The listing builds one solid part. Answer for the finished solid, in the listing's coordinates (mm). Face numbers are marked on the shaded views. A direction names the side the tool comes from. Coordinates: 2 decimals unless noted, no trailing zeros. Write each loop counter-clockwise with the first axis right and the second up, starting at its lowest first coordinate (ties: lowest second). Pieces come first, ordered by that corner, then holes. Notation, with made-up numbers: M 11,20 L 31,20 A4 cw 31,26 Z; hole C 3,58 d7. An arc over 180 degrees is marked long. Answer as a JSON object with one key per item and string values. Group by question number.
from build123d import *

# Parameters (mm, degrees)
SKETCH2_W           = 62
SKETCH2_H           = 49
BOSS_EXTRUDE2_DEPTH = 16
SKETCH3_W           = 60.436043862
SKETCH3_H           = 47.036060162
CUT_EXTRUDE2_DEPTH  = 15.492
SKETCH4_W           = 26
SKETCH4_H           = 26
CUT_EXTRUDE3_DEPTH  = 1.014
SKETCH6_W           = 11.5
SKETCH6_H           = 10
CUT_EXTRUDE4_DEPTH  = 1.014
FILLET3_R           = 1
SKETCH8_W           = 33.330843918
SKETCH8_H           = 11.266105729
BOSS_EXTRUDE3_DEPTH = 5.586
SKETCH9_W           = 2.5
SKETCH9_H           = 30.963135996
CUT_EXTRUDE5_DEPTH  = 13.714


with BuildPart() as part:
    # Sketch2 → Boss-Extrude2 (new body)
    with BuildSketch(Plane(origin=(0, 0, 0), x_dir=(1, 0, 0), z_dir=(0, 1, 0))):
        Rectangle(SKETCH2_W, SKETCH2_H)
    extrude(amount=BOSS_EXTRUDE2_DEPTH)

    # Sketch3 → Cut-Extrude2 (cut)
    with BuildSketch(Plane(origin=(0, 16, 0), x_dir=(1, 0, 0), z_dir=(0, 1, 0))):
        Rectangle(SKETCH3_W, SKETCH3_H)
    extrude(amount=-CUT_EXTRUDE2_DEPTH, mode=Mode.SUBTRACT)

    # Sketch4 → Cut-Extrude3 (cut)
    with BuildSketch(Plane.XZ):
        with Locations((0, 9.5)):
            Rectangle(SKETCH4_W, SKETCH4_H)
    extrude(amount=-CUT_EXTRUDE3_DEPTH, mode=Mode.SUBTRACT)

    # Sketch6 → Cut-Extrude4 (cut)
    with BuildSketch(Plane(origin=(0, 0, -24.5), x_dir=(-1, 0, 0), z_dir=(0, 0, -1))):
        with Locations((-16.25, 10.9998)):
            Rectangle(SKETCH6_W, SKETCH6_H)
    extrude(amount=-CUT_EXTRUDE4_DEPTH, mode=Mode.SUBTRACT)

    # Fillet3
    fillet3_edges = [part.edges().sort_by_distance(p)[0] for p in [
        (31, 8, 24.5),
        (-31, 8, 24.5),
        (-31, 8, -24.5),
        (31, 8, -24.5),
    ]]
    fillet(fillet3_edges, radius=FILLET3_R)

    # Sketch8 → Boss-Extrude3 (add)
    with BuildSketch(Plane.ZY.offset(31)):
        with Locations((0, 7.613654272)):
            Rectangle(SKETCH8_W, SKETCH8_H)
    boss_extrude3 = extrude(amount=BOSS_EXTRUDE3_DEPTH)

    # Sketch9 → Cut-Extrude5 (cut)
    with BuildSketch(Plane(origin=(0, 13.246707136, 0), x_dir=(1, 0, 0), z_dir=(0, 1, 0))):
        with Locations((-34.442433929, 0)):
            Rectangle(SKETCH9_W, SKETCH9_H)
    cut_extrude5 = extrude(amount=-CUT_EXTRUDE5_DEPTH, mode=Mode.SUBTRACT)

    # Mirror1: Boss-Extrude3, Cut-Extrude5 across plane
    add(boss_extrude3.mirror(Plane(origin=(0, 0, 0), x_dir=(0, 0, 1), z_dir=(1, 0, 0))))
    add(cut_extrude5.mirror(Plane(origin=(0, 0, 0), x_dir=(0, 0, 1), z_dir=(1, 0, 0))), mode=Mode.SUBTRACT)


solid = part.part
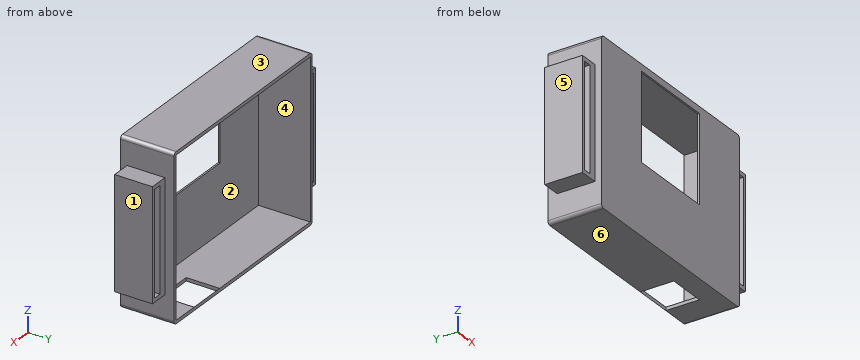
Item 1: Flat-ended cylindrical pins translate along their axes: pin 1 Ø4 at (x, z) = (14.5, -1.5) entering from +Y; pin 2 Ø3 at (x, y) = (-33, 5) entering from +Z; pin 3 Ø3 at (x, z) = (34, -8) entering from +Y; pin 4 Ø4 at (y, z) = (13.5, -4.5) entering from +X. Find the tip coordinate at first contact, or state that the pin passes through.
Item 2: Consider L1, parallel to X at y = 10.25, z = 10; L2, parallel to X at y = 1, z = 10; L3, parallel to Z at x = -8, y = 6.75. Determine where each line is inside the solid, lowest interval first. Write a range as from..to.
Item 3: A cutting plane is placed at C-C, the plane z = -5. Write down the section's boundary in (x, y), and give its area (3 significant figures).
Item 4: A tool of negligible diameter and unlimited length cuts with its end or side. For the marked faces 1 and 2, from which of +Z, -Z, +X, -X, +Y, -Y can it reach the whole face along a straight path? Write none if from no direction.
Item 5: For a pull along Z with two mould halves and no side action, classify the marked faces 3, 4, 5 and 6 as +Z half, -Z half, draft (parallel to the pull), parting line (faces both ways), or undercut.
Item 6: A cutting plane is placed at B-B, the plane y = 3. Write down the section's boundary in (x, z).
Item 7: A cutting plane is placed at D-D, the plane y = 12. State how many separate pieces and enclosed holes the cut face has, and give its area (3 significant figures).
Answer:
{
 "1": {"pin 1": "y = 0.51", "pin 2": "z = 16.67", "pin 3": "y = 13.25", "pin 4": "x = 36.59"},
 "2": {"L1": "-36.59..-35.69, -33.19..-30.22, 30.22..33.19, 35.69..36.59", "L2": "-31..-30.22, 30.22..31", "L3": "-24.5..-23.52, 23.52..24.5"},
 "3": {"outline": "M -36.59,1.98 L -35.69,1.98 L -35.69,13.25 L -36.59,13.25 Z; M -33.19,1.98 L -31,1.98 L -31,0 L 31,0 L 31,1.98 L 33.19,1.98 L 33.19,13.25 L 31,13.25 L 31,16 L 30.22,16 L 30.22,0.51 L -30.22,0.51 L -30.22,16 L -31,16 L -31,13.25 L -33.19,13.25 Z; M 35.69,1.98 L 36.59,1.98 L 36.59,13.25 L 35.69,13.25 Z", "area": "125 mm2"},
 "4": {"face 1": "+Z, -Z, +X, +Y, -Y", "face 2": "+Y"},
 "5": {"face 3": "+Z half", "face 4": "undercut", "face 5": "draft", "face 6": "-Z half"},
 "6": {"outline": "M -36.59,-16.67 L -31,-16.67 L -31,-23.5 A1 ccw -30,-24.5 L 30,-24.5 A1 ccw 31,-23.5 L 31,-16.67 L 36.59,-16.67 L 36.59,16.67 L 31,16.67 L 31,23.5 A1 ccw 30,24.5 L -30,24.5 A1 ccw -31,23.5 L -31,16.67 L -36.59,16.67 Z; hole M -35.69,-15.48 L -33.19,-15.48 L -33.19,15.48 L -35.69,15.48 Z; hole M -30.22,-23.52 L 30.22,-23.52 L 30.22,23.52 L -30.22,23.52 Z; hole M 33.19,-15.48 L 35.69,-15.48 L 35.69,15.48 L 33.19,15.48 Z"},
 "7": {"separate pieces": "1", "enclosed holes": "2", "area": "401 mm2"}
}
